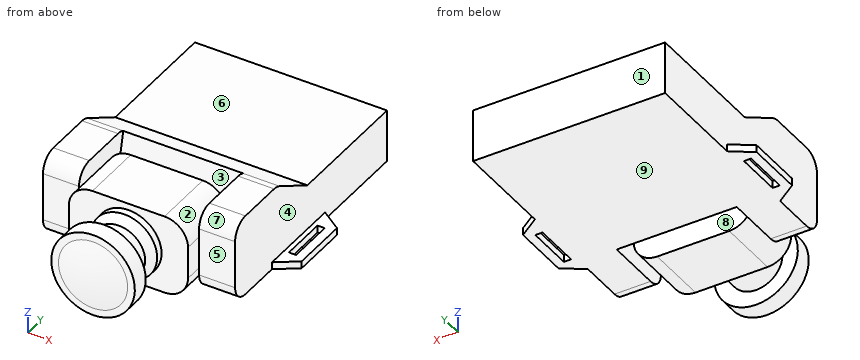
from build123d import *

# Parameters (mm, degrees)
F1_DEPTH  = 20
F3_DEPTH  = 17
F5_DEPTH  = 25
F7_DEPTH  = 1.5
F11_DEPTH = 13
F13_DEPTH = 42.1


with BuildPart() as f1:
    # F0 (on Right) → F1 (new body, symmetric)
    with BuildSketch(Plane.YZ):
        with BuildLine():
            Line((25.75, 0), (25.75, 11))
            Line((25.75, 11), (-1.25, 11))
            Line((-1.25, 11), (-10.75, 16.5254688627))
            ThreePointArc((-10.75, 16.5254688627), (-11.5984192745, 16.8792855028), (-12.5096983153, 17))
            Line((-12.5096983153, 17), (-22.25, 17))
            ThreePointArc((-22.25, 17), (-24.7248737342, 15.9748737342), (-25.75, 13.5))
            Line((-25.75, 13.5), (-25.75, 3.5))
            ThreePointArc((-25.75, 3.5), (-24.7248737342, 1.0251262658), (-22.25, 0))
            Line((-22.25, 0), (25.75, 0))
        make_face()
    extrude(amount=F1_DEPTH, both=True)

    # F2 (on face) → F3 (cut, through all)
    with BuildSketch(Plane.XY.offset(17)):
        Polygon((0, -12.5096983153), (-12.5, -12.5096983153), (-12.5, -25.75), (0, -25.75), (12.5, -25.75), (12.5, -12.5096983153), align=None)
    extrude(amount=-F3_DEPTH, mode=Mode.SUBTRACT)

    # F4 (on face) → F5 (cut, through all)
    with BuildSketch(Plane.YZ.offset(-12.5)):
        Polygon((-10.75, 0), (-12.5096983153, 8.5), (-12.5096983153, 0), align=None)
        with BuildLine():
            Line((-12.5096983153, 8.5), (-10.75, 16.5254688627))
            ThreePointArc((-10.75, 16.5254688627), (-11.5984192745, 16.8792855028), (-12.5096983153, 17))
            Line((-12.5096983153, 17), (-12.5096983153, 8.5))
        make_face()
    extrude(amount=F5_DEPTH, mode=Mode.SUBTRACT)

    # F6 (on face) → F7 (join)
    with BuildSketch(Plane(origin=(0, 0, 0), x_dir=(1, 0, 0), z_dir=(0, 0, -1))):
        Polygon((-24.33, -1.75), (-20, -4.75), (-20, 13.25), (-24.33, 10.25), (-24.33, 4.25), align=None)
        Polygon((-22.47, 4.25), (-22.47, 9.1), (-20.97, 9.1), (-20.97, 4.25), (-20.97, -0.6), (-22.47, -0.6), align=None, mode=Mode.SUBTRACT)
    extrude(amount=-F7_DEPTH)

    # F8: F1 across plane


with BuildPart() as f1_1:
    add(f1.part)
    add(f1.part.mirror(Plane.YZ))



with BuildPart() as f11:
    # F10 (on offset) → F11 (new body)
    with BuildSketch(Plane.XZ.offset(29.35)):
        with BuildLine():
            Line((0, 16.5254688627), (-7.5, 16.5254688627))
            ThreePointArc((-7.5, 16.5254688627), (-10.9648232278, 15.0902920905), (-12.4, 11.6254688627))
            Line((-12.4, 11.6254688627), (-12.4, 4.9))
            ThreePointArc((-12.4, 4.9), (-10.9648232278, 1.4351767722), (-7.5, 0))
            Line((-7.5, 0), (0, 0))
            Line((0, 0), (7.5, 0))
            ThreePointArc((7.5, 0), (10.9648232278, 1.4351767722), (12.4, 4.9))
            Line((12.4, 4.9), (12.4, 11.6254688627))
            ThreePointArc((12.4, 11.6254688627), (10.9648232278, 15.0902920905), (7.5, 16.5254688627))
            Line((7.5, 16.5254688627), (0, 16.5254688627))
        make_face()
    extrude(amount=-F11_DEPTH)


with BuildPart() as f1_2:
    add(f1_1.part)

    add(f11.part)  # F13 merges F11
    # F12 (on face) → F13 (join, through all)
    with BuildSketch(Plane(origin=(0, -16.35, 0), x_dir=(-1, 0, 0), z_dir=(0, 1, 0))):
        Polygon((0, 8.9999999979), (-5, 8.9999999979), (-5, 8.4999999979), (-5, 7.9999999979), (0, 7.9999999979), (5, 7.9999999979), (5, 8.4999999979), (5, 8.9999999979), align=None)
    extrude(amount=F13_DEPTH)

    # F14 (on Right) → F15 (revolve)
    with BuildSketch(Plane.YZ):
        with BuildLine():
            Line((-29.35, 4.9), (-29.35, 8.2627344313))
            Line((-29.35, 8.2627344313), (-41.35, 8.2627344313))
            Line((-41.35, 8.2627344313), (-42.85, 8.2627344313))
            ThreePointArc((-42.85, 8.2627344313), (-42.4710169679, 4.5854392297), (-41.35, 1.0627344313))
            Line((-41.35, 1.0627344313), (-41.35, -0.4372655687))
            Line((-41.35, -0.4372655687), (-37.65, -0.4372655687))
            Line((-37.65, -0.4372655687), (-37.65, 2.7627344313))
            Line((-37.65, 2.7627344313), (-32.65, 2.7627344313))
            Line((-32.65, 2.7627344313), (-30.85, 1.3627344313))
            Line((-30.85, 1.3627344313), (-29.35, 1.3627344313))
            Line((-29.35, 1.3627344313), (-29.35, 4.9))
        make_face()
    revolve(axis=Axis((0, -35.35, 8.2627344313), (0, -1, 0)))


solid = f1_2.part
Design review of the part built by this model. Coordinates are the model's own, in mm. Face numbers are marked on the shaded views. A direction names the side the tool comes from. Give positions to 0.01 mm unless a question says otherwise; leave off trailing zeros. Order: outer loops, then holes, each group sorted by start corner. A loop starts at its lowest first (then second) coordinate and runs counter-clockwise, first axis right, second up.
1. To check wall thickness, follow L1, parallel to X at y = -3, z = 0.5; L2, parallel to Y at x = 6, z = 10.25; L3, parallel to Y at x = 6, z = 11.5. State the ranges of each line that lie inside material, in increasing order.
Solution:
L1: x = -24.33 to -22.47, -20.97 to 20.97, 22.47 to 24.33
L2: y = -41.71 to -37.65, -31.6 to -16.35, -12.13 to 25.75
L3: y = -41.51 to -37.65, -30.96 to -16.35, -11.85 to -2.11
2. Add section D-D, the plane y = 9. State the section outline as (x, z) points, then the cut area to 3 significant figures.
Solution:
outline: (-20, 0) - (20, 0) - (20, 11) - (-20, 11) - close
area: 440 mm2
3. Mouldability with a two-part tool opening along X and no side actions: class the marked faces 1, 2, 3 and 4 as +X half, -X half, draft (parallel to the pull), parting line (faces both ways), or undercut.
Solution:
face 1: draft
face 2: undercut
face 3: undercut
face 4: +X half
4. Add section C-C, the plane x = 10. State the section outline as (y, z) points, then the cut area to 3 significant figures.
Solution:
outline: (-29.35, 0.69) - (-16.35, 0.69) - (-16.35, 15.84) - (-29.35, 15.84) - close; (-12.51, 8.5) - (-10.75, 0) - (25.75, 0) - (25.75, 11) - (-1.25, 11) - (-10.75, 16.53) - close
area: 639 mm2
5. Add section B-B, the plane y = -7. State the section outline as (x, z) points.
Solution:
outline: (-24.33, 0) - (-22.47, 0) - (-22.47, 1.5) - (-24.33, 1.5) - close; (-20.97, 0) - (20.97, 0) - (20.97, 1.5) - (20, 1.5) - (20, 14.34) - (-20, 14.34) - (-20, 1.5) - (-20.97, 1.5) - close; (22.47, 0) - (24.33, 0) - (24.33, 1.5) - (22.47, 1.5) - close
6. For pin 1 Ø3 at (x, y) = (12.5, 8.5) entering from -Z; pin 2 Ø3 at (x, y) = (-2.5, -14) entering from +Z; pin 3 Ø5 at (x, z) = (1, 5.5) entering from -Y, all flat-tipped, find the tip position at first contact; note any pin that passes through.
Solution:
pin 1: stops at z = 0
pin 2: stops at z = 9
pin 3: stops at y = -42.84
7. Tool access review of the marked faces 5, 6, 7, 8 and 9: name each direction out of +Z, -Z, +X, -X, +Y, -Y from which nothing blocks a thin tool from reaching the whole face with its end or side.
Solution:
face 5: +Z, -Z, +X, -Y
face 6: +Z, +X, -X, +Y
face 7: +Z, +X, -Y
face 8: none
face 9: -Z, +X, -X, +Y
8. Add section A-A, the plane x = 17.5. State the section outline as (y, z) points, then the cut area to 3 significant figures.
Solution:
outline: (-25.75, 3.5) arc R3.5 ccw to (-22.25, 0) - (25.75, 0) - (25.75, 11) - (-1.25, 11) - (-10.75, 16.53) arc R3.5 ccw to (-12.51, 17) - (-22.25, 17) arc R3.5 ccw to (-25.75, 13.5) - close
area: 677 mm2
